```python
from build123d import *

# Parameters (mm, degrees)
F0_R     = 32.25
F0_R_2   = 1.2
F0_R_3   = 26.5
F0_R_4   = 1.225
F1_DEPTH = 5
F2_DEPTH = 5.9
F3_R     = 0.5
F4_R     = 0.5


with BuildPart() as f1:
    # F0 (on Top) → F1 (new body)
    with BuildSketch(Plane.XY):
        Circle(F0_R)
        with Locations((0, -30)):
            Circle(F0_R_2, mode=Mode.SUBTRACT)
        Circle(F0_R_3, mode=Mode.SUBTRACT)
        with Locations((0, 29.5)):
            Circle(F0_R_4, mode=Mode.SUBTRACT)
    extrude(amount=F1_DEPTH)

    # F0 (on Top) → F2 (join)
    with BuildSketch(Plane.XY):
        Circle(F0_R)
        with Locations((0, -30)):
            Circle(F0_R_2, mode=Mode.SUBTRACT)
        Circle(F0_R_3, mode=Mode.SUBTRACT)
        with Locations((0, 29.5)):
            Circle(F0_R_4, mode=Mode.SUBTRACT)
    extrude(amount=F2_DEPTH)

    # F3
    f3_edges = [f1.edges().sort_by_distance(p)[0] for p in [
        (-26.5, 0, 0),
        (-32.25, 0, 0),
        (-32.25, 0, 5.9),
    ]]
    fillet(f3_edges, radius=F3_R)

    # F4
    f4_edges = [f1.edges().sort_by_distance(p)[0] for p in [
        (-26.5, 0, 5.9),
        (-32.25, 0, 5.4),
    ]]
    fillet(f4_edges, radius=F4_R)


solid = f1.part
```
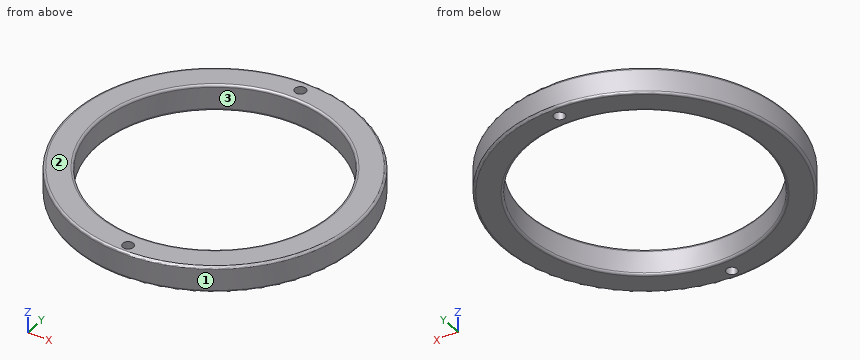
Design review of the part built by this model. Coordinates are the model's own, in mm. Face numbers are marked on the shaded views. Coordinates: 2 decimals unless noted, no trailing zeros. Loops run counter-clockwise (first coordinate to the right, second up) from the corner with the lowest first, then second, coordinate; pieces in that order, holes last. Notation, with made-up numbers: (89, 40.25) - (125, 40.25) arc R13 cw to (125, 58.25) - close; hole circle Ø2 at (65, 50.25). An arc over 180 degrees is marked (long way). Use CSV: the item, a comma, the result in double quotes. Start each with the question number.
1) For pin 1 Ø1.5 at (y, z) = (3, 1) entering from -X, flat-tipped, find the tip position at first contact; note if it passes through.
2) The part is to be moulded in two halves that separate along Y. For the marked faces 1, 2 and 3, say which applies: +Y half, -Y half, draft (parallel to the pull), parting line (faces both ways), or undercut.
3) Wall thickness on L1, parallel to Y at x = 0, z = 1.4 (3 decimals); L2, parallel to Y at x = -1, z = 3.5; L3, parallel to X at y = -21.5, z = 2.95: over which ranges is each line inside the solid? List them lowest first. Write a range as from..to.
4) Consider section B-B on x = 0. Write out the cut boundary in (y, z) (3 decimals), then the cut area to 3 significant figures.
5) Consider section A-A on y = 0. Write out the cut boundary in (x, z), then the cut area to 3 significant figures.
6) Consider section C-C on z = 2.5. Write out the cut boundary in (x, y) (3 decimals).
Geometry says:
1,pin 1,"x = -32.17"
2,face 1,"parting line"
2,face 2,"draft"
2,face 3,"undercut"
3,L1,"-32.25..-31.2, -28.8..-26.5, 26.5..28.275, 30.725..32.25"
3,L2,"-32.23..-30.66, -29.34..-26.48, 26.48..28.79, 30.21..32.23"
3,L3,"-24.04..-15.49, 15.49..24.04"
4,outline,"(-32.25, 0.5) arc R0.5 ccw to (-31.75, 0) - (-31.2, 0) - (-31.2, 5.9) - (-31.75, 5.9) arc R0.5 ccw to (-32.25, 5.4) - close; (-28.8, 0) - (-27, 0) arc R0.5 ccw to (-26.5, 0.5) - (-26.5, 5.4) arc R0.5 ccw to (-27, 5.9) - (-28.8, 5.9) - close; (26.5, 0.5) arc R0.5 ccw to (27, 0) - (28.275, 0) - (28.275, 5.9) - (27, 5.9) arc R0.5 ccw to (26.5, 5.4) - close; (30.725, 0) - (31.75, 0) arc R0.5 ccw to (32.25, 0.5) - (32.25, 5.4) arc R0.5 ccw to (31.75, 5.9) - (30.725, 5.9) - close"
4,area,"38.8 mm^2"
5,outline,"(-32.25, 0.5) arc R0.5 ccw to (-31.75, 0) - (-27, 0) arc R0.5 ccw to (-26.5, 0.5) - (-26.5, 5.4) arc R0.5 ccw to (-27, 5.9) - (-31.75, 5.9) arc R0.5 ccw to (-32.25, 5.4) - close; (26.5, 0.5) arc R0.5 ccw to (27, 0) - (31.75, 0) arc R0.5 ccw to (32.25, 0.5) - (32.25, 5.4) arc R0.5 ccw to (31.75, 5.9) - (27, 5.9) arc R0.5 ccw to (26.5, 5.4) - close"
5,area,"67.4 mm^2"
6,outline,"circle Ø64.5 at (0, 0); hole circle Ø53 at (0, 0); hole circle Ø2.45 at (0, 29.5); hole circle Ø2.4 at (0, -30)"
